Geometry: final body of the model. Coordinates: model frame, mm. Give positions to 0.01 mm unless a question says otherwise; leave off trailing zeros. Write each loop counter-clockwise with the first axis right and the second up, starting at its lowest first coordinate (ties: lowest second). Pieces come first, ordered by that corner, then holes. Notation, with made-up numbers: M 88.25,30.25 L 96.25,30.25 A14 ccw 96.25,43.25 Z; hole C 11.25,44.25 d5. An arc over 180 degrees is marked long. Answer as a JSON object with one key per item and string values.
from build123d import *

# Parameters (mm, degrees)
F0_W     = 609.6
F0_H     = 406.4
F1_DEPTH = 9.525
F2_W     = 9.525
F2_H     = 406.4
F3_DEPTH = 25.4
F4_W     = 600.075
F4_H     = 406.4
F4_W_2   = 9.525
F5_DEPTH = 9.525
F6_W     = 609.6
F6_H     = 44.45
F7_DEPTH = 9.525
F8_W     = 609.6
F8_H     = 44.45
F9_DEPTH = 9.525


# Not quite as in the source:
# - a length typed as a fraction of an inch, garbled in the dataset ("3 / 203.2 mm" for 3/8 in), is restored


with BuildPart() as f1:
    # F0 (on Front) → F1 (new body)
    with BuildSketch(Plane.XZ):
        Rectangle(F0_W, F0_H)
    extrude(amount=F1_DEPTH)

    # F2 (on face) → F3 (join)
    with BuildSketch(Plane(origin=(0, 0, 0), x_dir=(-1, 0, 0), z_dir=(0, 1, 0))):
        with Locations((-300.0375, 0)):
            Rectangle(F2_W, F2_H)
        with Locations((300.0375, 0)):
            Rectangle(F2_W, F2_H)
    extrude(amount=F3_DEPTH)

    # F4 (on face) → F5 (join)
    with BuildSketch(Plane(origin=(0, 25.4, 0), x_dir=(-1, 0, 0), z_dir=(0, 1, 0))):
        with Locations((4.7625, 0)):
            Rectangle(F4_W, F4_H)
        with Locations((-300.0375, 0)):
            Rectangle(F4_W_2, F4_H)
    extrude(amount=F5_DEPTH)

    # F6 (on face) → F7 (join)
    with BuildSketch(Plane(origin=(0, 0, -203.2), x_dir=(1, 0, 0), z_dir=(0, 0, -1))):
        with Locations((0, -12.7)):
            Rectangle(F6_W, F6_H)
    extrude(amount=F7_DEPTH)

    # F8 (on face) → F9 (join)
    with BuildSketch(Plane.XY.offset(203.2)):
        with Locations((0, 12.7)):
            Rectangle(F8_W, F8_H)
    extrude(amount=F9_DEPTH)


solid = f1.part
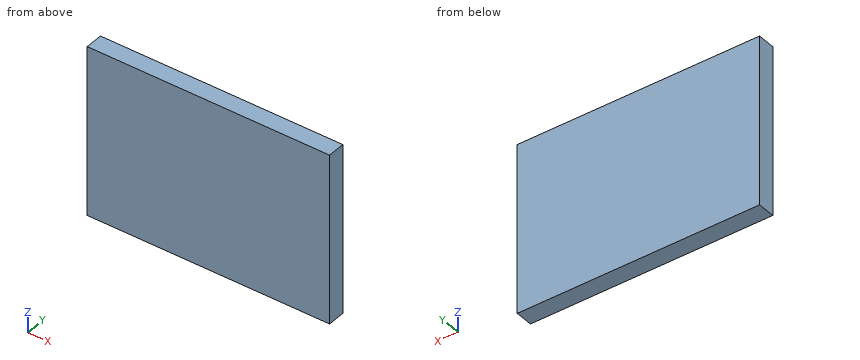
1) Cut plane B-B on y = 16.5. Return loops of the section in (x, z) (3 decimals).
Geometry check:
{"outline": "M -304.8,-212.725 L 304.8,-212.725 L 304.8,212.725 L -304.8,212.725 Z; hole M -295.275,-203.2 L 295.275,-203.2 L 295.275,203.2 L -295.275,203.2 Z"}
2) Cut plane A-A on z = 77. Return loops of the section in (x, y) (3 decimals).
Geometry check:
{"outline": "M -304.8,-9.525 L 304.8,-9.525 L 304.8,34.925 L -304.8,34.925 Z; hole M -295.275,0 L 295.275,0 L 295.275,25.4 L -295.275,25.4 Z"}
3) Line query: line 1 (Y direction, x = 66, z = -122.5) (3 decimals); line 2 (Z direction, x = 247, y = 9.5) (3 decimals); line 3 (X direction, y = 3.5, z = -130) (3 decimals). Output: solid intervals per line, ascending. Write a range as from..to.
Geometry check:
{"line 1": "y = -9.525..0, 25.4..34.925", "line 2": "z = -212.725..-203.2, 203.2..212.725", "line 3": "x = -304.8..-295.275, 295.275..304.8"}
